Could you check a few things on this model? Use its own coordinates, in mm. Face numbers are marked on the shaded views. A direction names the side the tool comes from. Coordinates: 2 decimals unless noted, no trailing zeros. Loops run counter-clockwise (first coordinate to the right, second up) from the corner with the lowest first, then second, coordinate; pieces in that order, holes last. Notation, with made-up numbers: M 34.5,22 L 69.5,22 A38 cw 69.5,60 Z; hole C -2.5,35.5 d2. An arc over 180 degrees is marked long. Use one line per item in the form item = value. Start each with the question number.
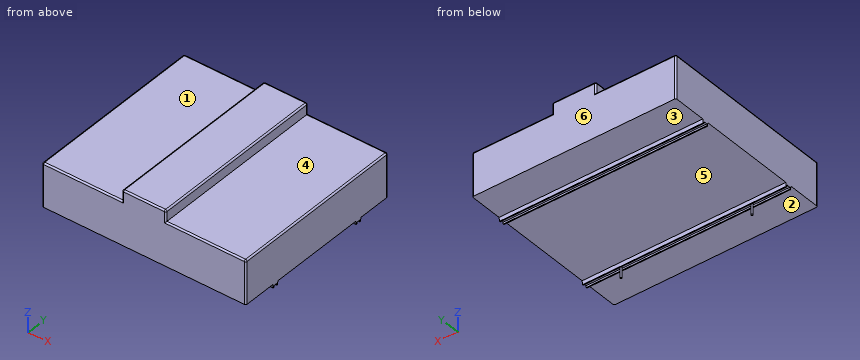
```python
from build123d import *

# Parameters (mm, degrees)
F1_DEPTH = 622.3
F2_R     = 10.16
F4_DEPTH = 1422.4
F5_R     = 6.35
F6_DEPTH = 76.2


with BuildPart() as f1:
    # F0 (on Front) → F1 (new body, symmetric)
    with BuildSketch(Plane.XZ):
        Polygon((711.2, -152.4), (711.2, 152.4), (152.4, 152.4), (152.4, 75.2325318336), (-152.4, 75.2325318336), (-152.4, 152.4), (-711.2, 152.4), (-711.2, -152.4), align=None)
        Polygon((152.4, 75.2325318336), (152.4, 152.4), (152.4, 229.5674681664), (-152.4, 229.5674681664), (-152.4, 152.4), (-152.4, 75.2325318336), align=None)
    extrude(amount=F1_DEPTH, both=True)

    # F2
    f2_edges = [f1.edges().sort_by_distance(p)[0] for p in [
        (711.2, 0, 152.4),
        (431.8, -622.3, 152.4),
        (711.2, -622.3, 0),
        (431.8, 622.3, 152.4),
        (711.2, 622.3, 0),
        (0, 622.3, 229.567468),
        (152.4, 622.3, 190.983734),
        (152.4, 0, 229.567468),
        (-152.4, 622.3, 190.983734),
        (-152.4, 0, 229.567468),
        (-431.8, 622.3, 152.4),
        (-711.2, 622.3, 0),
        (-711.2, 0, 152.4),
        (-711.2, -622.3, 0),
        (-431.8, -622.3, 152.4),
        (-152.4, -622.3, 190.983734),
        (0, -622.3, 229.567468),
        (152.4, -622.3, 190.983734),
    ]]
    fillet(f2_edges, radius=F2_R)

    # F3 (on face) → F4 (join)
    with BuildSketch(Plane.YZ.offset(711.2)):
        Polygon((-342.265, -152.4), (-386.715, -152.4), (-383.54, -177.8), (-377.5456, -177.8), (-377.5456, -165.1), (-351.4344, -165.1), (-351.4344, -177.8), (-345.44, -177.8), align=None)
        Polygon((386.715, -152.3999997139), (342.265, -152.3999997139), (345.44, -177.7999997139), (351.4344, -177.7999997139), (351.4344, -165.0999997139), (377.5456, -165.0999997139), (377.5456, -177.7999997139), (383.54, -177.7999997139), align=None)
    extrude(amount=-F4_DEPTH)

    # F5 (on face) → F6 (join)
    with BuildSketch(Plane(origin=(0, 0, -165.1), x_dir=(1, 0, 0), z_dir=(0, 0, -1))):
        with Locations((457.2, 364.49)):
            Circle(F5_R)
        with Locations((-457.2, 364.49)):
            Circle(F5_R)
    extrude(amount=F6_DEPTH)


solid = f1.part
```
Item 1: For the marked faces 1, 2 and 3, which set-ups out of +Z, -Z, +X, -X, +Y, -Y let a thin tool reach every point of the face, with its end or its side?
Item 2: I want a section at A-A (y = -490.5). Write out the boundary of the cut face in (x, z).
Item 3: Please list where these lines run through material, in increasing order: line 1 along Z through (x, y) = (416, 434); line 2 along Z through (x, y) = (-402, -360).
Item 4: Thinking about a two-plate mould opening in Y: for the marked faces 4, 5 and 6, which applies, pulls with the +Y half, pulls with the -Y half, needs draft (parallel to the pull), parting line crosses it, or undercut?
Item 5: I want a section at C-C (z = -208). Write out the boundary of the cut face in (x, y), plus the area to 3 significant figures.
Item 6: I'm going to push flat-ended pins straight in: P1, Ø5, axis at x = -43, y = -380, coming from the -Z side; P2, Ø13, axis at x = 73.5, y = 360.5, coming from the -Z side; P3, Ø4, axis at x = -151, z = -171, coming from the -Y side. Where does each tip first touch, or does it pass through?
Item 7: I want a section at B-B (x = -383). Write out the boundary of the cut face in (y, z) (3 decimals).
Worked answers:
q1.face_1 = +Z, -X, +Y, -Y
q1.face_2 = -Z, +X, -X, -Y
q1.face_3 = -Z, +X, -X, +Y
q2.outline = M -711.2,-152.4 L 711.2,-152.4 L 711.2,142.24 A10.16 ccw 701.04,152.4 L 152.4,152.4 L 152.4,219.41 A10.16 ccw 142.24,229.57 L -142.24,229.57 A10.16 ccw -152.4,219.41 L -152.4,152.4 L -701.04,152.4 A10.16 ccw -711.2,142.24 Z
q3.line_1 = -152.4 to 152.4
q3.line_2 = -165.1 to 152.4
q4.face_4 = needs draft
q4.face_5 = undercut
q4.face_6 = pulls with the +Y half
q5.outline = C -457.2,-364.49 d12.7; C 457.2,-364.49 d12.7
q5.area = 253 mm²
q6.P1 = -177.8
q6.P2 = -165.1
q6.P3 = -384.64
q7.outline = M -622.3,-152.4 L -386.715,-152.4 L -383.54,-177.8 L -377.546,-177.8 L -377.546,-165.1 L -351.434,-165.1 L -351.434,-177.8 L -345.44,-177.8 L -342.265,-152.4 L 342.265,-152.4 L 345.44,-177.8 L 351.434,-177.8 L 351.434,-165.1 L 377.546,-165.1 L 377.546,-177.8 L 383.54,-177.8 L 386.715,-152.4 L 622.3,-152.4 L 622.3,142.24 A10.16 ccw 612.14,152.4 L -612.14,152.4 A10.16 ccw -622.3,142.24 Z
